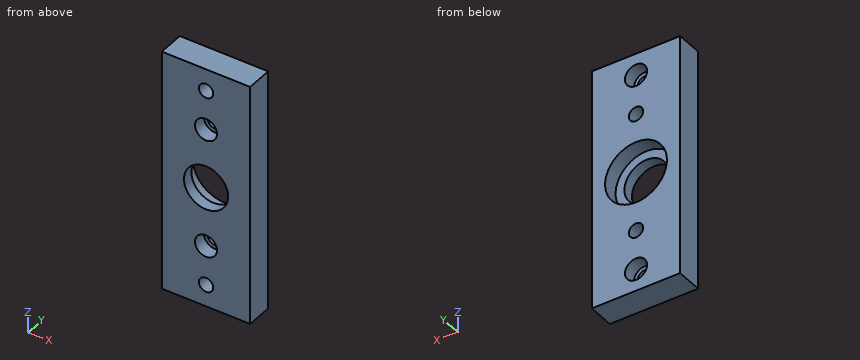
from build123d import *

# Parameters (mm, degrees)
F0_W     = 40
F0_H     = 110
F0_R     = 3.25
F0_R_2   = 10
F1_DEPTH = 12
F2_R     = 5
F3_DEPTH = 6
F4_R     = 5
F5_DEPTH = 6
F6_R     = 14
F6_R_2   = 10
F7_DEPTH = 7


with BuildPart() as f1:
    # F0 (on Front) → F1 (new body)
    with BuildSketch(Plane.XZ):
        with Locations((20, 55)):
            Rectangle(F0_W, F0_H)
        with Locations((20, 10)):
            Circle(F0_R, mode=Mode.SUBTRACT)
        with Locations((20, 28)):
            Circle(F0_R, mode=Mode.SUBTRACT)
        with Locations((20, 55)):
            Circle(F0_R_2, mode=Mode.SUBTRACT)
        with Locations((20, 82)):
            Circle(F0_R, mode=Mode.SUBTRACT)
        with Locations((20, 100)):
            Circle(F0_R, mode=Mode.SUBTRACT)
    extrude(amount=F1_DEPTH)

    # F2 (on face) → F3 (cut)
    with BuildSketch(Plane.XZ.offset(12)):
        with Locations((20, 82)):
            Circle(F2_R)
        with Locations((20, 28)):
            Circle(F2_R)
    extrude(amount=-F3_DEPTH, mode=Mode.SUBTRACT)

    # F4 (on face) → F5 (cut)
    with BuildSketch(Plane(origin=(0, 0, 0), x_dir=(-1, 0, 0), z_dir=(0, 1, 0))):
        with Locations((-20, 100)):
            Circle(F4_R)
        with Locations((-20, 10)):
            Circle(F4_R)
    extrude(amount=-F5_DEPTH, mode=Mode.SUBTRACT)

    # F6 (on face) → F7 (cut)
    with BuildSketch(Plane(origin=(0, 0, 0), x_dir=(-1, 0, 0), z_dir=(0, 1, 0))):
        with Locations((-20, 55)):
            Circle(F6_R)
        with Locations((-20, 55)):
            Circle(F6_R_2, mode=Mode.SUBTRACT)
    extrude(amount=-F7_DEPTH, mode=Mode.SUBTRACT)


solid = f1.part
Design review of the part built by this model. Coordinates are the model's own, in mm. Round coordinates to 2 decimals unless told otherwise and drop trailing zeros. Loops run counter-clockwise (first coordinate to the right, second up) from the corner with the lowest first, then second, coordinate; pieces in that order, holes last. Notation, with made-up numbers: (-26, 41) - (24, 41) arc R16 cw to (24, 65) - close; hole circle Ø11 at (7, 8). An arc over 180 degrees is marked (long way). One line per item, written item: value. Start each with the question number.
1) Insertion check: pin 1 Ø14 at (x, z) = (16.5, 55.5) entering from +Y; pin 2 Ø5 at (x, z) = (21, 29) entering from -Y; pin 3 Ø3 at (x, z) = (18.5, 7.5) entering from +Y; pin 4 Ø4 at (x, z) = (20, 82) entering from -Y. Each pin has a flat end and moves straight along its axis. Give the tip position at first contact, or say it passes through.
2) To check wall thickness, follow L1, parallel to Z at x = 20, y = -10.6; L2, parallel to Z at x = 20, y = -5; L3, parallel to X at y = -9, z = 10. State the ranges of each line that lie inside material, in increasing order. Write a range as from..to.
3) Consider section A-A on y = -9.75. Give the boundary of the cut face in (x, z).
4) Consider section D-D on z = 55. Give the boundary of the cut face in (x, y).
5) Consider section C-C on x = 20. Give the number of separate pieces and of enclosed holes in the cut face, then the cut area to 3 significant figures.
6) Consider section B-B on z = 100. Give the boundary of the cut face in (x, y).
Reported:
1. pin 1: stops at y = -7
1. pin 2: stops at y = -6
1. pin 3: stops at y = -6
1. pin 4: passes through
2. L1: z = 0..6.75, 13.25..23, 33..45, 65..77, 87..96.75, 103.25..110
2. L2: z = 0..5, 15..24.75, 31.25..41, 69..78.75, 85.25..95, 105..110
2. L3: x = 0..16.75, 23.25..40
3. outline: (0, 0) - (40, 0) - (40, 110) - (0, 110) - close; hole circle Ø20 at (20, 55); hole circle Ø10 at (20, 28); hole circle Ø10 at (20, 82); hole circle Ø6.5 at (20, 10); hole circle Ø6.5 at (20, 100)
4. outline: (0, -12) - (10, -12) - (10, -7) - (6, -7) - (6, 0) - (0, 0) - close; (30, -12) - (40, -12) - (40, 0) - (34, 0) - (34, -7) - (30, -7) - close
5. separate pieces: 6
5. enclosed holes: 0
5. area: 628 mm^2
6. outline: (0, -12) - (16.75, -12) - (16.75, -6) - (15, -6) - (15, 0) - (0, 0) - close; (23.25, -12) - (40, -12) - (40, 0) - (25, 0) - (25, -6) - (23.25, -6) - close
